from build123d import *

# Parameters (mm, degrees)
SKETCH1_R               = 66.04
BOSS_EXTRUDE1_DEPTH     = 12.7
CUT_EXTRUDE1_DEPTH      = 95.254194602
CUT_EXTRUDE1_DEPTH_BACK = 95.254194602
SKETCH2_R               = 3.175
SKETCH4_R               = 4.826
CUT_EXTRUDE2_DEPTH      = 95.254194602


with BuildPart() as part:
    # Sketch1 → Boss-Extrude1 (new body)
    with BuildSketch(Plane(origin=(0, 0, 0), x_dir=(1, 0, 0), z_dir=(0, 1, 0))):
        with Locations(Location((0, 0, 0), (0, 0, 270))):
            Circle(SKETCH1_R)
    extrude(amount=BOSS_EXTRUDE1_DEPTH)

    # Sketch2 → Cut-Extrude1 (cut, two sides: drawn at the far end of the back side and taken through both)
    with BuildSketch(Plane(origin=(0, 12.7, 0), x_dir=(1, 0, 0), z_dir=(0, 1, 0)).offset(-CUT_EXTRUDE1_DEPTH_BACK)):
        with Locations(Location((-44.214813621, 15.875, 0), (0, 0, 270))):
            Circle(SKETCH2_R)
        with Locations(Location((-44.214813621, -15.875, 0), (0, 0, 270))):
            Circle(SKETCH2_R)
        with Locations(Location((44.214813621, -15.875, 0), (0, 0, 270))):
            Circle(SKETCH2_R)
        with Locations(Location((44.214813621, 15.875, 0), (0, 0, 270))):
            Circle(SKETCH2_R)
    extrude(amount=CUT_EXTRUDE1_DEPTH + CUT_EXTRUDE1_DEPTH_BACK, mode=Mode.SUBTRACT)

    # Sketch4 → Cut-Extrude2 (cut, through all)
    with BuildSketch(Plane.XZ):
        with Locations(Location((0, 0, 0), (0, 0, 270))):
            Circle(SKETCH4_R)
    extrude(amount=-CUT_EXTRUDE2_DEPTH, mode=Mode.SUBTRACT)


solid = part.part
The listing builds one solid part. Answer for the finished solid, in the listing's coordinates (mm). Coordinates: 2 decimals unless noted, no trailing zeros. Order: outer loops, then holes, each group sorted by start corner. A loop starts at its lowest first (then second) coordinate and runs counter-clockwise, first axis right, second up.
Q1. A cutting plane is placed at A-A, the plane z = 0. Write down the section's boundary in (x, y).
Q2. A cutting plane is placed at B-B, the plane x = 0. Write down the section's boundary in (y, z).
Q3. Consider line 1 (Z direction, x = -47, y = 2.25); line 2 (X direction, y = 6, z = -17.5); line 3 (X direction, y = 7.5, z = -4). Determine where each line is inside the solid, lowest interval first.
Q4. A cutting plane is placed at D-D, the plane x = 23.5. Write down the section's boundary in (y, z).
Q5. A cutting plane is placed at C-C, the plane y = 9.5. Write down the section's boundary in (x, z) (3 decimals), and give its area (3 significant figures).
Q6. For a pull along Z with two mould halves and no side action, classify faces 1 (the face through (41.115, 6.261, -16.563)), 2 (the face through (-40.18, 6.26, -52.41)), 3 (the face through (-14, 0, -1)) as pulls with the +Z half, pulls with the -Z half, needs draft (parallel to the pull), parting line crosses it, or undercut.
Q7. Given P1, Ø5, axis at x = 44.21, z = -15.88, coming from the +Y side; P2, Ø3, axis at y = 9.5, z = 32.5, coming from the +X side; P3, Ø1.5, axis at y = 3.5, z = -33.5, coming from the +X side; P4, Ø2, axis at x = 14, y = 11, coming from the +Z side, each flat-ended and moving along its own axis, determine where each tip first touches the part or whether it passes through.
Answers follow:
1. outline: (-66.04, 0) - (-4.83, 0) - (-4.83, 12.7) - (-66.04, 12.7) - close; (4.83, 0) - (66.04, 0) - (66.04, 12.7) - (4.83, 12.7) - close
2. outline: (0, -66.04) - (12.7, -66.04) - (12.7, -4.83) - (0, -4.83) - close; (0, 4.83) - (12.7, 4.83) - (12.7, 66.04) - (0, 66.04) - close
3. line 1: z = -46.39 to -17.4, -14.35 to 14.35, 17.4 to 46.39
3. line 2: x = -63.68 to -46.94, -41.49 to 41.49, 46.94 to 63.68
3. line 3: x = -65.92 to -2.7, 2.7 to 65.92
4. outline: (0, -61.72) - (12.7, -61.72) - (12.7, 61.72) - (0, 61.72) - close
5. outline: circle Ø132.08 at (0, 0); hole circle Ø6.35 at (-44.215, -15.875); hole circle Ø6.35 at (-44.215, 15.875); hole circle Ø9.652 at (0, 0); hole circle Ø6.35 at (44.215, -15.875); hole circle Ø6.35 at (44.215, 15.875)
5. area: 13,500 mm2
6. face 1: undercut
6. face 2: parting line crosses it
6. face 3: needs draft
7. P1: passes through
7. P2: stops at x = 58.31
7. P3: stops at x = 57.35
7. P4: stops at z = 64.75
